Design review of the part built by this model. Coordinates are the model's own, in mm. Face numbers are marked on the shaded views. A direction names the side the tool comes from. Coordinates: 2 decimals unless noted, no trailing zeros. Loops run counter-clockwise (first coordinate to the right, second up) from the corner with the lowest first, then second, coordinate; pieces in that order, holes last.
Q1. Add section B-B on y = -9. Give the boundary of the cut face in (x, z).
Q2. Machinability: for the marked faces 1 and 2, which of the approach directions +Z, -Z, +X, -X, +Y, -Y give a long, thin tool a straight path to every point of the face, cutting with its end or side? Answer none if there is none.
Q3. Add section A-A on z = -12. Give the boundary of the cut face in (x, y).
Q4. Add section C-C on z = 0. Give the boundary of the cut face in (x, y).
Q5. Wall thickness on probe 1 along X at (y, z) = (-7.5, -9); probe 2 along Y at (x, z) = (-6.5, -7.75); probe 3 along Y at (x, z) = (39.55, 0): over which ranges is each line inside the solid? List them lowest first.
Q6. Add section D-D on x = 11.5. Give the boundary of the cut face in (y, z), and give its area (3 significant figures).
Q7. For P1, Ø2.5, axis at y = 0, z = -15.5, coming from the -X side; P2, Ø3, axis at y = 1.5, z = 6, coming from the -X side; P3, Ø0.6, axis at x = 45, y = -0.5, coming from the -Z side, all flat-tipped, find the tip position at first contact; note any pin that passes through.
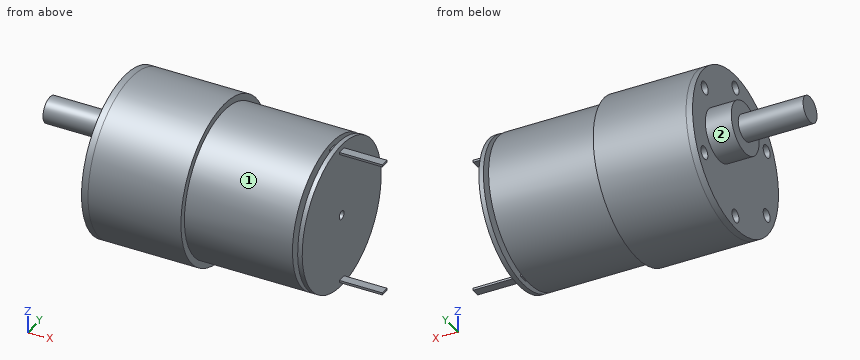
```python
from build123d import *

# Parameters (mm, degrees)
SKETCH1_R                      = 17
BOSS_EXTRUDE1_DEPTH            = 1.05
SKETCH2_W                      = 0.5
SKETCH2_H                      = 2
POLES_DEPTH                    = 1.2
POLES_DEPTH_BACK               = 11
SKETCH3_R                      = 1.5
BOSS_EXTRUDE3_DEPTH            = 1.2
SKETCH5_R                      = 17
BOSS_EXTRUDE5_DEPTH            = 25
SKETCH6_R                      = 18.5
REDUCTUR_DEPTH                 = 21.5
SKETCH35_R                     = 18.5
ENDPLATE_DEPTH                 = 1.5
SKETCH36_R                     = 6
BOSS_EXTRUDE25_DEPTH           = 6
F_3_1_3_1_DIAMETER_HOLE1_D     = 6
F_3_1_3_1_DIAMETER_HOLE1_DEPTH = 2.2
F_2_0_2_DIAMETER_HOLE1_D       = 2
F_2_0_2_DIAMETER_HOLE1_DEPTH   = 2.25
F_3_0MM_1_D                    = 3
F_3_0MM_1_DEPTH                = 7.5
F_3_0MM_1_TIP                  = 0.901290929
SKETCH_1_R                     = 3
EXTRUDE_1_DEPTH                = 21


with BuildPart() as part:
    # Sketch1 → Boss-Extrude1 (new body)
    with BuildSketch(Plane(origin=(41.25, 0, 0), x_dir=(0, 0, -1), z_dir=(1, 0, 0))):
        Circle(SKETCH1_R)
    extrude(amount=-BOSS_EXTRUDE1_DEPTH)

    # Sketch2 → Poles (add, two sides)
    with BuildSketch(Plane.ZY.offset(-40.2)) as poles_sk:
        with Locations((15.5, 0)):
            Rectangle(SKETCH2_W, SKETCH2_H)
        with Locations((-15.5, 0)):
            Rectangle(SKETCH2_W, SKETCH2_H)
    extrude(amount=POLES_DEPTH)
    extrude(poles_sk.sketch, amount=-POLES_DEPTH_BACK)

    # Sketch3 → Boss-Extrude3 (add)
    with BuildSketch(Plane.ZY.offset(-40.2)):
        Circle(SKETCH3_R)
    extrude(amount=BOSS_EXTRUDE3_DEPTH)

    # Sketch5 → Boss-Extrude5 (add)
    with BuildSketch(Plane(origin=(39, 0, 0), x_dir=(0, 0, -1), z_dir=(1, 0, 0))):
        Circle(SKETCH5_R)
    extrude(amount=-BOSS_EXTRUDE5_DEPTH)

    # Sketch6 → Reductur (add)
    with BuildSketch(Plane(origin=(14, 0, 0), x_dir=(0, 0, -1), z_dir=(1, 0, 0))):
        Circle(SKETCH6_R)
    extrude(amount=-REDUCTUR_DEPTH)

    # Sketch35 → Endplate (add)
    with BuildSketch(Plane.ZY.offset(7.5)):
        Circle(SKETCH35_R)
    extrude(amount=ENDPLATE_DEPTH)

    # Sketch36 → Boss-Extrude25 (add)
    with BuildSketch(Plane.ZY.offset(9)):
        with Locations((0, 7)):
            Circle(SKETCH36_R)
    extrude(amount=BOSS_EXTRUDE25_DEPTH)

    # Ø3.1 (3.1) Diameter Hole1
    with Locations(Plane.ZY.offset(15)):
        with Locations((0, 7)):
            Hole(F_3_1_3_1_DIAMETER_HOLE1_D / 2, depth=F_3_1_3_1_DIAMETER_HOLE1_DEPTH)

    # Ø2.0 (2) Diameter Hole1
    with Locations(Plane(origin=(41.25, 0, 0), x_dir=(0, 0, -1), z_dir=(1, 0, 0))):
        with Locations((0, 0)):
            Hole(F_2_0_2_DIAMETER_HOLE1_D / 2, depth=F_2_0_2_DIAMETER_HOLE1_DEPTH)

    # Ø3.0mm 定位孔1
    with Locations(Plane(origin=(-9, 0, -15.5), x_dir=(0, 0, -1), z_dir=(-1, 0, 0))):
        with Locations((0, 0), (-7.75, -13.423393759), (-23.50507477, -13.272858695), (-31, 0), (-23.25, 13.423393759), (-7.75, 13.423393759)):
            Hole(F_3_0MM_1_D / 2, depth=F_3_0MM_1_DEPTH)
            with Locations((0, 0, -(F_3_0MM_1_DEPTH + F_3_0MM_1_TIP / 2))):  # 118° drill point
                Cone(0, F_3_0MM_1_D / 2, F_3_0MM_1_TIP, mode=Mode.SUBTRACT)

    # 草圖1 → 填料-伸長1 (add)
    with BuildSketch(Plane.ZY.offset(9)):
        with Locations((0, 7)):
            Circle(SKETCH_1_R)
    extrude(amount=EXTRUDE_1_DEPTH)


solid = part.part
```
Entries:
1. outline: (-9, -16.16) - (14, -16.16) - (14, -14.42) - (39, -14.42) - (39, 14.42) - (14, 14.42) - (14, 16.16) - (-9, 16.16) - close; (40.2, -14.42) - (41.25, -14.42) - (41.25, 14.42) - (40.2, 14.42) - close
2. face 1: +X
2. face 2: -X
3. outline: (-9, -14.08) - (14, -14.08) - (14, -12.04) - (39, -12.04) - (39, 12.04) - (14, 12.04) - (14, 14.08) - (-9, 14.08) - close; (40.2, -12.04) - (41.25, -12.04) - (41.25, 12.04) - (40.2, 12.04) - close
4. outline: (-30, 4) - (-15, 4) - (-15, 1) - (-9, 1) - (-9, -18.5) - (14, -18.5) - (14, -17) - (39, -17) - (39, -1.5) - (40.2, -1.5) - (40.2, -17) - (41.25, -17) - (41.25, -1) - (39, -1) - (39, 1) - (41.25, 1) - (41.25, 17) - (40.2, 17) - (40.2, 1.5) - (39, 1.5) - (39, 17) - (14, 17) - (14, 18.5) - (-9, 18.5) - (-9, 13) - (-15, 13) - (-15, 10) - (-30, 10) - close
5. probe 1: x = -9 to 39, 40.2 to 41.25
5. probe 2: y = -16.8 to -14.92, -11.92 to 11.92, 14.92 to 16.8
5. probe 3: y = -1.5 to -1, 1 to 1.5
6. outline: circle Ø37 at (0, 0)
6. area: 1,080 mm2
7. P1: stops at x = -1.35
7. P2: stops at x = -9
7. P3: stops at z = -15.75
